Design review of the part built by this model. Coordinates are the model's own, in mm. A direction names the side the tool comes from. Give positions to 0.01 mm unless a question says otherwise; leave off trailing zeros. Order: outer loops, then holes, each group sorted by start corner. A loop starts at its lowest first (then second) coordinate and runs counter-clockwise, first axis right, second up.
```python
from build123d import *

# Parameters (mm, degrees)
SKETCH1_R           = 1.1
BOSS_EXTRUDE1_DEPTH = 5
BOSS_EXTRUDE2_DEPTH = 9
FILLET1_R           = 15
SKETCH3_R           = 1
CUT_EXTRUDE1_DEPTH  = 16
FILLET2_R           = 3
SKETCH4_R           = 1.9
CUT_EXTRUDE2_DEPTH  = 1
FILLET3_R           = 1.5
FILLET4_R           = 0.5


with BuildPart() as part:
    # Sketch1 → Boss-Extrude1 (new body)
    with BuildSketch(Plane.XY):
        with BuildLine():
            ThreePointArc((0, 4.5), (-4.5, 0), (0, -4.5))
            Line((0, -4.5), (50, -4.5))
            Line((50, -4.5), (50, 4.5))
            Line((50, 4.5), (0, 4.5))
        make_face()
        Circle(SKETCH1_R, mode=Mode.SUBTRACT)
    extrude(amount=BOSS_EXTRUDE1_DEPTH)

    # Sketch2 → Boss-Extrude2 (add)
    with BuildSketch(Plane(origin=(0, 4.5, 0), x_dir=(1, 0, 0), z_dir=(0, 1, 0))):
        Polygon((50.5, 2), (60, 2), (60, 5.5), (50, 5.5), (50, 0), (50, -5), (50, -10.5), (60, -10.5), (60, -7), (50.5, -7), align=None)
    extrude(amount=-BOSS_EXTRUDE2_DEPTH)

    # Fillet1
    # the kernel refuses this fillet: 15 mm, written as the material it adds along each edge
    with BuildSketch(Plane(origin=(50, -4.5, 0), x_dir=(0, 0, -1), z_dir=(0, 1, 0))) as fillet1_piece_1:
        with BuildLine():
            CenterArc((15, 11.608186766), FILLET1_R, 180, 50.703519761)
            Line((0, 11.608186766), (-0.3, 11.608186766))
            Line((-0.3, 11.608186766), (-0.3, 0))
            Line((-0.3, 0), (0, -0.3))
            ThreePointArc((0, -0.3), (2.75, -0.3), (5.31, -0.232163735))
            Line((5.31, -0.232163735), (5.5, 0))
        make_face()
    extrude(amount=9)
    with BuildSketch(Plane(origin=(50, -4.5, 5), x_dir=(0, 0, 1), z_dir=(0, 1, 0))) as fillet1_piece_2:
        with BuildLine():
            CenterArc((15, -11.608186766), FILLET1_R, 129.296480239, 50.703519761)
            Line((0, -11.608186766), (-0.3, -11.608186766))
            Line((-0.3, -11.608186766), (-0.3, 0))
            Line((-0.3, 0), (0, 0.3))
            ThreePointArc((0, 0.3), (2.75, 0.3), (5.31, 0.232163735))
            Line((5.31, 0.232163735), (5.5, 0))
        make_face()
    extrude(amount=9)

    # Sketch3 → Cut-Extrude1 (cut)
    with BuildSketch(Plane.XY.offset(10.5)):
        with Locations((56, 0)):
            Circle(SKETCH3_R)
    extrude(amount=-CUT_EXTRUDE1_DEPTH, mode=Mode.SUBTRACT)

    # Fillet2
    fillet2_edges = [part.edges().sort_by_distance(p)[0] for p in [
        (60, 4.5, 8.75),
        (60, 4.5, -3.75),
        (60, -4.5, 8.75),
        (60, -4.5, -3.75),
    ]]
    fillet(fillet2_edges, radius=FILLET2_R)

    # Sketch4 → Cut-Extrude2 (cut)
    with BuildSketch(Plane.XY.offset(10.5)):
        with Locations((56, 0)):
            Circle(SKETCH4_R)
    extrude(amount=-CUT_EXTRUDE2_DEPTH, mode=Mode.SUBTRACT)

    # Fillet3
    fillet3_edges = [part.edges().sort_by_distance(p)[0] for p in [
        (50.5, 0, 7),
        (50.5, 0, -2),
    ]]
    fillet(fillet3_edges, radius=FILLET3_R)

    # Fillet4
    fillet4_edges = [part.edges().sort_by_distance(p)[0] for p in [
        (55, 0, -2),
    ]]
    fillet(fillet4_edges, radius=FILLET4_R)


solid = part.part
```
1. Take a section at C-C (z = 4). State the section outline as (x, y) points, then the cut area to 3 significant figures.
Recorded:
outline: (0, -4.5) - (50.5, -4.5) - (50.5, 4.5) - (0, 4.5) arc R4.5 ccw to start; hole circle Ø2.2 at (0, 0)
area: 483 mm2
2. Machinability: for faces 1 (the face through (17, 0, 5)), 2 (the face through (54.1, 0.08, 10.01)), 3 (the face through (50.95, -0.06, -1.57)), which of the approach directions +Z, -Z, +X, -X, +Y, -Y give a long, thin tool a straight path to every point of the face, cutting with its end or side? Answer none if there is none.
Recorded:
face 1: +Z, -X, +Y, -Y
face 2: +Z
face 3: +X, +Y, -Y
3. Draft analysis for pull direction X (two halves, no side actions). For faces 4 (the face through (-4.5, 0.1, 2.5)), 5 (the face through (55, 0, -4)), 6 (the face through (17, 0, 0)), state which applies: pulls with the +X half, pulls with the -X half, needs draft (parallel to the pull), parting line crosses it, or undercut.
Recorded:
face 4: pulls with the -X half
face 5: undercut
face 6: needs draft
4. Take a section at D-D (y = -2.75). State the section outline as (x, z) points.
Recorded:
outline: (-3.56, 0) - (38.39, 0) arc R15 cw to (50, -5.5) - (59.73, -5.5) - (59.73, -2) - (52, -2) arc R1.5 cw to (50.5, -0.5) - (50.5, 5.5) arc R1.5 cw to (52, 7) - (59.73, 7) - (59.73, 10.5) - (50, 10.5) arc R15 cw to (38.39, 5) - (-3.56, 5) - close
5. Take a section at B-B (x = 56). State the section outline as (y, z) points, then the cut area to 3 significant figures.
Recorded:
outline: (-4.5, -5.5) - (-1, -5.5) - (-1, -2.5) arc R0.5 ccw to (-1.5, -2) - (-4.5, -2) - close; (-4.5, 7) - (-1, 7) - (-1, 9.5) - (-1.9, 9.5) - (-1.9, 10.5) - (-4.5, 10.5) - close; (1, -5.5) - (4.5, -5.5) - (4.5, -2) - (1.5, -2) arc R0.5 ccw to (1, -2.5) - close; (1, 7) - (4.5, 7) - (4.5, 10.5) - (1.9, 10.5) - (1.9, 9.5) - (1, 9.5) - close
area: 47.1 mm2
6. For pin 1 (3 mm diameter, centred on x = 56, y = 0, fed in from +Z); pin 2 (2 mm diameter, centred on x = 11.5, y = -1.5, fed in from -Z); pin 3 (2.5 mm diameter, centred on x = 0, y = 0, fed in from +Z), all flat-tipped, find the tip position at first contact; note any pin that passes through.
Recorded:
pin 1: stops at z = 9.5
pin 2: stops at z = 0
pin 3: stops at z = 5
7. For line 1 along Y through (x, z) = (56, -4.55); line 2 along Z through (x, y) = (55, 2.75); line 3 along Z through (x, y) = (6.5, 3.75), list the stretches that pass through material, from the lowest coordinate up.
Recorded:
line 1: y = -4.5 to -1, 1 to 4.5
line 2: z = -5.5 to -2, 7 to 10.5
line 3: z = 0 to 5
8. Take a section at A-A (y = 0). State how many separate pieces and enclosed holes the cut face has, then the cut area to 3 significant figures.
Recorded:
separate pieces: 4
enclosed holes: 0
area: 360 mm2
